Input: part model. Units: mm. Frame: model coordinates. Give positions to 0.01 mm unless a question says otherwise; leave off trailing zeros. Order: outer loops, then holes, each group sorted by start corner. A loop starts at its lowest first (then second) coordinate and runs counter-clockwise, first axis right, second up.
```python
from build123d import *

# Parameters (mm, degrees)
STOCK_TORSO_FRONT_PLATE_1_START       = -1.5875
STOCK_TORSO_FRONT_PLATE_1_OUTLINE_W   = 96.34
STOCK_TORSO_FRONT_PLATE_1_OUTLINE_H   = 174.5
STOCK_TORSO_FRONT_PLATE_1_OUTLINE_W_2 = 3.4925
STOCK_TORSO_FRONT_PLATE_1_OUTLINE_H_2 = 10.25
STOCK_TORSO_FRONT_PLATE_1_OUTLINE_R   = 1.45
STOCK_TORSO_FRONT_PLATE_1_DEPTH       = 3.175
CUT_EXTRUDE1_DEPTH                    = 158.576741701
LPATTERN1_COUNT                       = 16
LPATTERN1_PITCH                       = 10
FILLET1_R                             = 1


# Read off the part's stored shape, not the designer's step: Stock-torso_front_plate-1
with BuildPart() as part:
    # Stock-torso_front_plate-1 outline → Stock-torso_front_plate-1 (new body)
    with BuildSketch(Plane.XY.offset(STOCK_TORSO_FRONT_PLATE_1_START)):
        with Locations((0, -62.75)):
            Rectangle(STOCK_TORSO_FRONT_PLATE_1_OUTLINE_W, STOCK_TORSO_FRONT_PLATE_1_OUTLINE_H)
        with Locations((-44.17, -141)):
            Rectangle(STOCK_TORSO_FRONT_PLATE_1_OUTLINE_W_2, STOCK_TORSO_FRONT_PLATE_1_OUTLINE_H_2, mode=Mode.SUBTRACT)
        with Locations((-44.17, -120)):
            Circle(STOCK_TORSO_FRONT_PLATE_1_OUTLINE_R, mode=Mode.SUBTRACT)
        with Locations((44.17, -141)):
            Rectangle(STOCK_TORSO_FRONT_PLATE_1_OUTLINE_W_2, STOCK_TORSO_FRONT_PLATE_1_OUTLINE_H_2, mode=Mode.SUBTRACT)
        with Locations((44.17, -120)):
            Circle(STOCK_TORSO_FRONT_PLATE_1_OUTLINE_R, mode=Mode.SUBTRACT)
        with Locations((-44.17, -40)):
            Circle(STOCK_TORSO_FRONT_PLATE_1_OUTLINE_R, mode=Mode.SUBTRACT)
        with Locations((-44.17, 0)):
            Rectangle(STOCK_TORSO_FRONT_PLATE_1_OUTLINE_W_2, STOCK_TORSO_FRONT_PLATE_1_OUTLINE_H_2, mode=Mode.SUBTRACT)
        with Locations((44.17, -40)):
            Circle(STOCK_TORSO_FRONT_PLATE_1_OUTLINE_R, mode=Mode.SUBTRACT)
        with Locations((44.17, 0)):
            Rectangle(STOCK_TORSO_FRONT_PLATE_1_OUTLINE_W_2, STOCK_TORSO_FRONT_PLATE_1_OUTLINE_H_2, mode=Mode.SUBTRACT)
    extrude(amount=STOCK_TORSO_FRONT_PLATE_1_DEPTH)

    # Sketch1 → Cut-Extrude1 (cut, symmetric)
    with BuildSketch(Plane.XY.offset(1.5875)):
        with BuildLine():
            Line((-25, 14.5), (25, 14.5))
            ThreePointArc((25, 14.5), (27.5, 12), (25, 9.5))
            Line((25, 9.5), (-25, 9.5))
            ThreePointArc((-25, 9.5), (-27.5, 12), (-25, 14.5))
        make_face()
    cut_extrude1 = extrude(amount=CUT_EXTRUDE1_DEPTH, both=True, mode=Mode.SUBTRACT)

    # LPattern1: Cut-Extrude1 ×16
    with Locations(*[(0, -i * LPATTERN1_PITCH, 0) for i in range(1, LPATTERN1_COUNT)]):
        add(cut_extrude1, mode=Mode.SUBTRACT)

    # Fillet1
    fillet1_edges = [part.edges().sort_by_distance(p)[0] for p in [
        (48.17, -150, 0),
        (-48.17, -150, 0),
        (-48.17, 24.5, 0),
        (48.17, 24.5, 0),
    ]]
    fillet(fillet1_edges, radius=FILLET1_R)


solid = part.part
```
1) Cut plane A-A (y = -3.5). Return the cut outline in (x, z), then the cut area to 3 significant figures.
2) Cut plane B-B (y = -108). Return the cut outline in (x, z).
3) Line query: probe 1 along Y at (x, z) = (44.17, 0.45) (3 decimals); probe 2 along X at (y, z) = (-2, -0.15); probe 3 along X at (y, z) = (-120, -0.6). Output: solid intervals per line, ascending.
4) Cut plane C-C (z = -0.1). Count the separate pieces of the cut face and the enclosed holes in it, then the cut area to 3 significant figures.
Geometry says:
1. outline: (-48.17, -1.59) - (-45.92, -1.59) - (-45.92, 1.59) - (-48.17, 1.59) - close; (-42.42, -1.59) - (42.42, -1.59) - (42.42, 1.59) - (-42.42, 1.59) - close; (45.92, -1.59) - (48.17, -1.59) - (48.17, 1.59) - (45.92, 1.59) - close
1. area: 284 mm2
2. outline: (-48.17, -1.59) - (-27.5, -1.59) - (-27.5, 1.59) - (-48.17, 1.59) - close; (27.5, -1.59) - (48.17, -1.59) - (48.17, 1.59) - (27.5, 1.59) - close
3. probe 1: y = -150 to -146.125, -135.875 to -121.45, -118.55 to -41.45, -38.55 to -5.125, 5.125 to 24.5
3. probe 2: x = -48.17 to -45.92, -42.42 to 42.42, 45.92 to 48.17
3. probe 3: x = -48.17 to -45.62, -42.72 to -26.5, 26.5 to 42.72, 45.62 to 48.17
4. separate pieces: 1
4. enclosed holes: 24
4. area: 12,300 mm2
